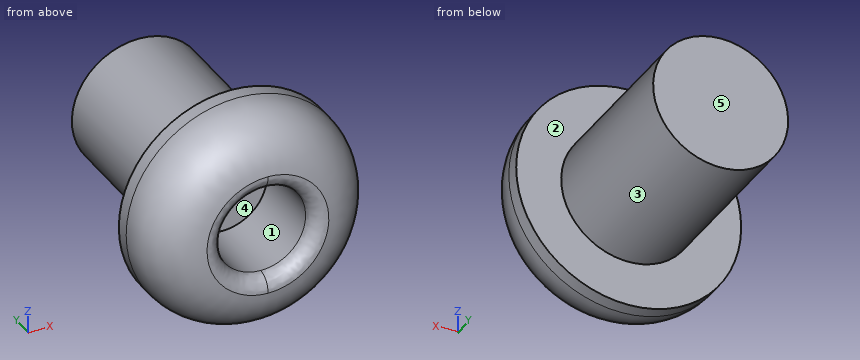
from build123d import *

# Parameters (mm, degrees)
SKETCH1_R                = 3.96875
SKETCH1_R_2              = 2.38125
BOSS_EXTRUDE2_DEPTH      = 2.54
BOSS_EXTRUDE3_DEPTH      = 6.35
BOSS_EXTRUDE3_DEPTH_BACK = 2.54
SKETCH2_R                = 2.38125
SKETCH3_R                = 1.5875
CUT_EXTRUDE1_DEPTH       = 3.175
FILLET1_R                = 2.032
FILLET2_R                = 0.508


with BuildPart() as part:
    # Sketch1 → Boss-Extrude2 (new body)
    with BuildSketch(Plane(origin=(0, 0, 0), x_dir=(1, 0, 0), z_dir=(0, 1, 0))):
        with Locations(Location((0, 0, 0), (0, 0, 270))):
            Circle(SKETCH1_R)
        with Locations(Location((0, 0, 0), (0, 0, 270))):
            Circle(SKETCH1_R_2, mode=Mode.SUBTRACT)
    extrude(amount=BOSS_EXTRUDE2_DEPTH)

    # Sketch2 → Boss-Extrude3 (add, two sides: drawn at the far end of the back side and taken through both)
    with BuildSketch(Plane(origin=(0, 2.54, 0), x_dir=(1, 0, 0), z_dir=(0, 1, 0)).offset(-BOSS_EXTRUDE3_DEPTH_BACK)):
        with Locations(Location((0, 0, 0), (0, 0, 270))):
            Circle(SKETCH2_R)
    extrude(amount=BOSS_EXTRUDE3_DEPTH + BOSS_EXTRUDE3_DEPTH_BACK)

    # Sketch3 → Cut-Extrude1 (cut)
    with BuildSketch(Plane(origin=(0, 0, 0), x_dir=(-1, 0, 0), z_dir=(0, -1, 0))):
        with Locations(Location((0, 0, 0), (0, 0, 90))):
            Circle(SKETCH3_R)
    extrude(amount=-CUT_EXTRUDE1_DEPTH, mode=Mode.SUBTRACT)

    # Fillet1
    fillet1_edges = [part.edges().sort_by_distance(p)[0] for p in [
        (0, 0, -3.96875),
    ]]
    fillet(fillet1_edges, radius=FILLET1_R)

    # Fillet2
    fillet2_edges = [part.edges().sort_by_distance(p)[0] for p in [
        (0, 0, 1.5875),
    ]]
    fillet(fillet2_edges, radius=FILLET2_R)


solid = part.part
Here's how the part is built. I have some questions about the finished solid (model axes, mm). Face numbers are marked on the shaded views. A direction names the side the tool comes from. Coordinates: 2 decimals unless noted, no trailing zeros. Loops run counter-clockwise (first coordinate to the right, second up) from the corner with the lowest first, then second, coordinate; pieces in that order, holes last.
1. I need wall thicknesses on L1, parallel to Y at x = -1.25, z = -1.75; L2, parallel to X at y = 1.4, z = 0; L3, parallel to X at y = 0.5, z = -0.75. Which ranges of each line are inside material? Lowest first, please.
2. For the marked faces 4 and 5, which set-ups out of +Z, -Z, +X, -X, +Y, -Y let a thin tool reach every point of the face, with its end or its side?
3. Imagine slicing it at A-A, the plane y = 4. Please give me the cut outline in (x, z).
4. For P1, Ø3, axis at y = 5, z = -1.5, coming from the +X side; P2, Ø2.5, axis at x = 0.5, z = 0.5, coming from the -Y side; P3, Ø2, axis at y = 1, z = 3, coming from the -X side; P4, Ø1, axis at x = 3, y = 6.5, coming from the +Z side, each with a flat end and sliding along its axis, tell me the tip position at first contact or that it passes through.
5. If we mould it in two halves opening along Z, with no side actions, what happens to the marked faces 1, 2 and 3? For each: pulls with the +Z half, pulls with the -Z half, needs draft (parallel to the pull), parting line crosses it, or undercut.
Taken from the geometry:
1. L1: y = 0.01 to 8.89
1. L2: x = -3.87 to -1.59, 1.59 to 3.87
1. L3: x = -3.18 to -1.4, 1.4 to 3.18
2. face 4: -Y
2. face 5: +Z, -Z, +X, -X, +Y
3. outline: circle Ø4.76 at (0, 0)
4. P1: stops at x = 2.38
4. P2: stops at y = 0.03
4. P3: stops at x = -3.26
4. P4: passes through
5. face 1: undercut
5. face 2: needs draft
5. face 3: parting line crosses it
